from build123d import *

# Parameters (mm, degrees)
F1_DEPTH = 72
F4_W     = 106.2124588788
F4_H     = 94.8871162292
F5_DEPTH = 47.4435581146
F7_DEPTH = 48


with BuildPart() as f1:
    # F0 (on Front) → F1 (new body, symmetric)
    with BuildSketch(Plane.XZ):
        with BuildLine():
            Line((-76.0368704796, -47.4435581146), (0, -47.4435581146))
            ThreePointArc((0, -47.4435581146), (47.4435581146, 0), (0, 47.4435581146))
            Line((0, 47.4435581146), (-76.0368704796, 47.4435581146))
            Line((-76.0368704796, 47.4435581146), (-76.0368704796, -47.4435581146))
        make_face()
    extrude(amount=F1_DEPTH, both=True)

    # F4 (on plane+point) → F5 (cut, through all)
    with BuildSketch(Plane.YZ.offset(47.4435581146)):
        with Locations((-18.8937705606, 0)):
            Rectangle(F4_W, F4_H)
    extrude(amount=-F5_DEPTH, mode=Mode.SUBTRACT)

    # F6 (on face) → F7 (cut)
    with BuildSketch(Plane.YZ):
        Polygon((-72, -27.6897922158), (34.2124588788, 47.4435581146), (-72, 47.4435581146), align=None)
    extrude(amount=-F7_DEPTH, mode=Mode.SUBTRACT)


solid = f1.part
Read the model definition and answer for the solid it produces. Units are mm, in the model's axes. A direction names the side the tool comes from. Round coordinates to 2 decimals unless told otherwise and drop trailing zeros. Order: outer loops, then holes, each group sorted by start corner. A loop starts at its lowest first (then second) coordinate and runs counter-clockwise, first axis right, second up.
1) The part is cut by section A-A on x = -36.5. Write down the section's boundary in (y, z), plus the area to 3 significant figures.
2) For faces 1 (the face through (-48, -31, 19)), 2 (the face through (-54, 15, 47.444)), 3 (the face through (0, -8, -10)), determine the directions among +Z, -Z, +X, -X, +Y, -Y from which every point of the face is accessible in a straight line to the end or side of a thin tool.
3) Straight lines are drawn through the part: L1, parallel to Y at x = 17.5, z = -23; L2, parallel to X at y = -21, z = -10; L3, parallel to X at y = -12, z = 18. For each, find the intervals that lie inside material, in ascending order.
4) The part is cut by section C-C on y = 15. Write down the section's boundary in (x, z).
5) Flat-ended cylindrical pins translate along their axes: pin 1 (22.5 mm diameter, centred on y = -22.5, z = 3, fed in from +X); pin 2 (1 mm diameter, centred on x = -46, z = 14, fed in from -Y). Find the tip coordinate at first contact, or state that the pin passes through.
6) The part is cut by section D-D on z = 28.5. Write down the section's boundary in (x, y).
7) The part is cut by section B-B on z = 0. Write down the section's boundary in (x, y), plus the area to 3 significant figures.
Resolved:
1. outline: (-72, -47.44) - (72, -47.44) - (72, 47.44) - (34.21, 47.44) - (-72, -27.69) - close
1. area: 9,670 mm2
2. face 1: +Z, +X, -Y
2. face 2: +Z, +X, -X, +Y, -Y
2. face 3: +Z, -Z, +X, -Y
3. L1: y = 34.21 to 72
3. L2: x = -76.04 to 0
3. L3: x = -76.04 to -48
4. outline: (-76.04, -47.44) - (0, -47.44) - (0, 33.85) - (-48, 33.85) - (-48, 47.44) - (-76.04, 47.44) - close
5. pin 1: stops at x = 0
5. pin 2: stops at y = -13.77
6. outline: (-76.04, -72) - (-48, -72) - (-48, 7.43) - (0, 7.43) - (0, 34.21) - (37.93, 34.21) - (37.93, 72) - (-76.04, 72) - close
7. outline: (-76.04, -72) - (-48, -72) - (-48, -32.86) - (0, -32.86) - (0, 34.21) - (47.44, 34.21) - (47.44, 72) - (-76.04, 72) - close
7. area: 10,900 mm2
